Drawing for the job (mm, zero at the part's lowest x, y, z). A direction names the side the tool comes from. Give positions to 0.01 mm unless a question says otherwise; leave off trailing zeros. Order: outer loops, then holes, each group sorted by start corner. A loop starts at its lowest first (then second) coordinate and runs counter-clockwise, first axis right, second up. Notation, with made-up numbers: M -40,-13.5 L -2,-13.5 A27 cw -2,6.5 Z; hole C 6,68 d9. An arc over 180 degrees is marked long. Answer as a JSON object with one key per item and string values.
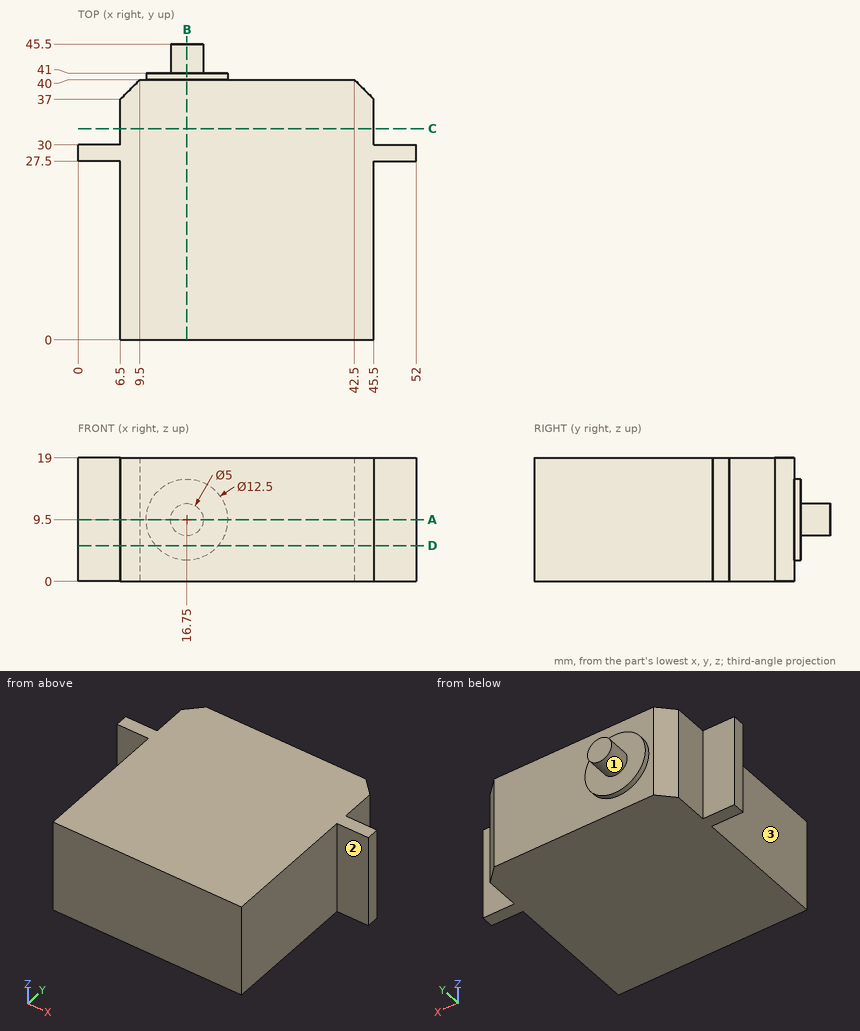
1. Cut at A-A on z = 9.5. Give the cut face in (x, y).
Worked answers:
{"outline": "M 0,27.5 L 6.5,27.5 L 6.5,0 L 45.5,0 L 45.5,27.5 L 52,27.5 L 52,30 L 45.5,30 L 45.5,37 L 42.5,40 L 23,40 L 23,41 L 19.25,41 L 19.25,45.5 L 14.25,45.5 L 14.25,41 L 10.5,41 L 10.5,40 L 9.5,40 L 6.5,37 L 6.5,30 L 0,30 Z"}
2. Cut at D-D on z = 5.5. Give the cut face in (x, y).
Worked answers:
{"outline": "M 0,27.5 L 6.5,27.5 L 6.5,0 L 45.5,0 L 45.5,27.5 L 52,27.5 L 52,30 L 45.5,30 L 45.5,37 L 42.5,40 L 21.55,40 L 21.55,41 L 11.95,41 L 11.95,40 L 9.5,40 L 6.5,37 L 6.5,30 L 0,30 Z"}
3. Cut at C-C on y = 32.5. Give the cut face in (x, z), plus the area to 3 significant figures.
Worked answers:
{"outline": "M 6.5,0 L 45.5,0 L 45.5,19 L 6.5,19 Z", "area": "741 mm^2"}
4. Which spindle directions (+Z, -Z, +X, -X, +Y, -Y) get a long thin tool onto all of the face, cutting with end or side? Do the marked faces 1, 2 and 3. Say none if no direction does.
Worked answers:
{"face 1": "+Y", "face 2": "+Z, -Z, +X, -Y", "face 3": "+Z, -Z, -X, -Y"}
5. Probe line 1 along Y through (x, z) = (10, 4); line 2 along X through (y, z) = (19, 3.75); line 3 along Y through (x, z) = (3, 8.5). List the from-to ranges inside material, lowest first.
Worked answers:
{"line 1": "y = 0 to 40", "line 2": "x = 6.5 to 45.5", "line 3": "y = 27.5 to 30"}
6. Cut at B-B on x = 16.75. Give the cut face in (y, z), plus the area to 3 significant figures.
Worked answers:
{"outline": "M 0,0 L 40,0 L 40,3.25 L 41,3.25 L 41,7 L 45.5,7 L 45.5,12 L 41,12 L 41,15.75 L 40,15.75 L 40,19 L 0,19 Z", "area": "795 mm^2"}
7. Pin check, flat tips, straight feed: P1, Ø2, axis at y = 32, z = 11, coming from the -X side; P2, Ø1.5, axis at x = 10.5, z = 15.5, coming from the +Y side; P3, Ø4, axis at x = 16, z = 17, coming from the +Y side; P4, Ø12, axis at x = 15, y = 9.5, coming from the -Z side. Stop position of each tip, or through.
Worked answers:
{"P1": "stops at x = 6.5", "P2": "stops at y = 40", "P3": "stops at y = 41", "P4": "stops at z = 0"}
